from build123d import *

# Parameters (mm, degrees)
BOSS_EXTRUDE1_DEPTH             = 10
F_5_0MM_DOWEL_HOLE1_D           = 5
F_5_0MM_DOWEL_HOLE1_CSINK_D     = 5.05
F_5_0MM_DOWEL_HOLE1_CSINK_ANGLE = 90
SKETCH5_W                       = 10
SKETCH5_H                       = 7.5
CUT_EXTRUDE1_DEPTH              = 20
SKETCH6_R                       = 7.5
CUT_EXTRUDE2_DEPTH              = 7.5
CHAMFER1_SIZE                   = 2
FILLET1_R                       = 1
F_5_0MM_DOWEL_HOLE2_D           = 5
F_5_0MM_DOWEL_HOLE2_DEPTH       = 10
F_5_0MM_DOWEL_HOLE2_TIP         = 1.502151548


with BuildPart() as part:
    # Sketch1 → Boss-Extrude1 (new body)
    with BuildSketch(Plane(origin=(0, 0, 0), x_dir=(1, 0, 0), z_dir=(0, 1, 0))):
        with BuildLine():
            Line((-5, 14.142135624), (-5, 22))
            Line((-5, 22), (-10, 22))
            Line((-10, 22), (-10, 11.180339887))
            ThreePointArc((-10, 11.180339887), (0, -15), (10, 11.180339887))
            Line((10, 11.180339887), (10, 22))
            Line((10, 22), (5, 22))
            Line((5, 22), (5, 14.142135624))
            ThreePointArc((5, 14.142135624), (0, 15), (-5, 14.142135624))
        make_face()
    extrude(amount=BOSS_EXTRUDE1_DEPTH)

    # Ø5.0mm Dowel Hole1 (through all)
    with Locations(Plane.ZY.offset(10)):
        with Locations((-18.5, 5)):
            CounterSinkHole(F_5_0MM_DOWEL_HOLE1_D / 2, F_5_0MM_DOWEL_HOLE1_CSINK_D / 2, counter_sink_angle=F_5_0MM_DOWEL_HOLE1_CSINK_ANGLE)

    # Sketch5 → Cut-Extrude1 (cut)
    with BuildSketch(Plane(origin=(0, 0, -22), x_dir=(-1, 0, 0), z_dir=(0, 0, -1))):
        with Locations((0, 3.75)):
            Rectangle(SKETCH5_W, SKETCH5_H)
    extrude(amount=-CUT_EXTRUDE1_DEPTH, mode=Mode.SUBTRACT)

    # Sketch6 → Cut-Extrude2 (cut)
    with BuildSketch(Plane.XZ):
        Circle(SKETCH6_R)
    extrude(amount=-CUT_EXTRUDE2_DEPTH, mode=Mode.SUBTRACT)

    # Chamfer1
    chamfer1_edges = [part.edges().sort_by_distance(p)[0] for p in [
        (0, 7.5, -15),
    ]]
    chamfer(chamfer1_edges, length=CHAMFER1_SIZE)

    # Fillet1
    fillet1_edges = [part.edges().sort_by_distance(p)[0] for p in [
        (-10, 0, -16.590169944),
        (-7.5, 0, -22),
        (-7.5, 10, -22),
        (10, 5, -22),
        (-10, 5, -22),
        (-10, 10, -16.590169944),
        (10, 10, -16.590169944),
        (7.5, 10, -22),
        (7.5, 0, -22),
        (10, 0, -16.590169944),
    ]]
    fillet(fillet1_edges, radius=FILLET1_R - 0.0001)  # a hair under: the kernel refuses the full size

    # Ø5.0mm Dowel Hole2
    with Locations(Plane(origin=(0, 0, 0), x_dir=(-1, 0, 0), z_dir=(0, -1, 0))):
        with Locations((-11.25, 0), (0, -11.25), (11.25, 0)):
            Hole(F_5_0MM_DOWEL_HOLE2_D / 2, depth=F_5_0MM_DOWEL_HOLE2_DEPTH)
            with Locations((0, 0, -(F_5_0MM_DOWEL_HOLE2_DEPTH + F_5_0MM_DOWEL_HOLE2_TIP / 2))):  # 118° drill point
                Cone(0, F_5_0MM_DOWEL_HOLE2_D / 2, F_5_0MM_DOWEL_HOLE2_TIP, mode=Mode.SUBTRACT)


solid = part.part
Geometry: final body of the model. Coordinates: model frame, mm. A direction names the side the tool comes from. Round coordinates to 2 decimals unless told otherwise and drop trailing zeros. Loops run counter-clockwise (first coordinate to the right, second up) from the corner with the lowest first, then second, coordinate; pieces in that order, holes last. Notation, with made-up numbers: M 42.5,-22.5 L 80.5,-22.5 A15 ccw 80.5,-11.5 Z; hole C 33.5,20 d3. An arc over 180 degrees is marked long. Put each result on its own line as item: value. Start each with the question number.
(1) Draft query along Z for faces 1 (the face through (8.752, 5.07, -0.11)), 2 (the face through (-7, 5, -22)), 3 (the face through (10, 5, -15)). Return one class per face: +Z half, -Z half, draft (parallel to the pull), parting line (faces both ways), or undercut.
(2) Material intervals for line 1 along Z through (x, y) = (0, 4); line 2 along Y through (x, z) = (6.3, -18.5); line 3 along Z through (x, y) = (-6, 5), sorted ascending. Write a range as [from, to].
(3) Section query B-B (x = 0). Return loops of the section in (y, z), then the cut area to 4 significant figures.
(4) Section query A-A (z = 0). Return loops of the section in (x, y).
(5) Set-up query: faces 4 (the face through (9.699, 0.285, -16.159)), 5 (the face through (0, 7.5, -3)), 6 (the face through (-5, 4, -14)). Return all of +Z, -Z, +X, -X, +Y, -Y with unobstructed straight access to the full face (end or side cutting, diameter ignored); none if empty.
(6) Contact query for flat-ended pins moving along their axis: pin 1 Ø5 at (y, z) = (7, 7.5) entering from -X; pin 2 Ø5 at (x, y) = (-3.5, 5.5) entering from +Z; pin 3 Ø5 at (y, z) = (6.5, -17.5) entering from +X. Output: stop coordinate, or through.
(7) Section query C-C (z = -18.5). Return loops of the section in (x, y) (3 decimals).
(8) Section query D-D (z = 11.25). Return loops of the section in (x, y).
Findings below:
1. face 1: undercut
1. face 2: -Z half
1. face 3: draft
2. line 1: z = [7.5, 8.75], [13.75, 15]
2. line 2: y = [0, 2.5], [7.5, 10]
2. line 3: z = [-22, -21], [-16, -4.5], [4.5, 13.75]
3. outline: M 0,7.5 L 7.5,7.5 L 7.5,-13 L 9.5,-15 L 10,-15 L 10,8.75 L 0,8.75 Z; M 0,13.75 L 10,13.75 L 10,15 L 0,15 Z
3. area: 79.25 mm2
4. outline: M -15,0 L -13.75,0 L -13.75,10 L -15,10 Z; M -8.75,0 L -7.5,0 L -7.5,7.5 L 7.5,7.5 L 7.5,0 L 8.75,0 L 8.75,10 L -8.75,10 Z; M 13.75,0 L 15,0 L 15,10 L 13.75,10 Z
5. face 4: -Z, +X, -Y
5. face 5: -Y
5. face 6: -Z, -Y
6. pin 1: stops at x = -14.14
6. pin 2: stops at z = 14.97
6. pin 3: stops at x = 10
7. outline: M -10,1 A1 ccw -9,0 L -5,0 L -5,2.5 L -9.975,2.5 L -10,2.475 Z; M -10,7.525 L -9.975,7.5 L -5,7.5 L -5,10 L -9,10 A1 ccw -10,9 Z; M 5,0 L 9,0 A1 ccw 10,1 L 10,2.5 L 5,2.5 Z; M 5,7.5 L 10,7.5 L 10,9 A1 ccw 9,10 L 5,10 Z
8. outline: M -9.92,0 L -2.5,0 L -2.5,10 L -9.92,10 Z; M 2.5,0 L 9.92,0 L 9.92,10 L 2.5,10 Z
